Input: part model. Units: mm. Frame: model coordinates. Face numbers are marked on the shaded views. A direction names the side the tool comes from. Round coordinates to 2 decimals unless told otherwise and drop trailing zeros. Loops run counter-clockwise (first coordinate to the right, second up) from the corner with the lowest first, then second, coordinate; pieces in that order, holes last. Notation, with made-up numbers: M 28,80 L 35,80 A23 cw 35,92 Z; hole C -10,-26 d1. An arc over 180 degrees is marked long. Use one line per item in the form item = value. Start each with the question number.
Q1. Section query D-D, the plane z = -23.5. Output: boundary loops of the cut face in (x, y), and give its area (3 significant figures).
Q2. Ray query, line 1 along Y through (x, z) = (-24.5, -28.5); line 2 along Z through (x, y) = (-24, -39.5); line 3 along X through (y, z) = (-79.5, -7). Return the intervals inside material, ascending.
Q3. Access query for the marked faces 1, 2 and 3. Directions: +Z, -Z, +X, -X, +Y, -Y. A direction counts if a zero-diameter tool reaches every point of the face in a straight line with its end or side. Return the directions, or none.
Q4. Section query A-A, the plane z = -34. Output: boundary loops of the cut face in (x, y).
Q5. First-contact query: P1, Ø1.5, axis at y = -70, z = -45, coming from the +X side; P2, Ø20.5, axis at x = -74, z = -34, coming from the -Y side; P3, Ø10, axis at x = -48, z = -21, coming from the +Y side. Flat tips, straight axial feed; report the tip coordinate or a pass-through.
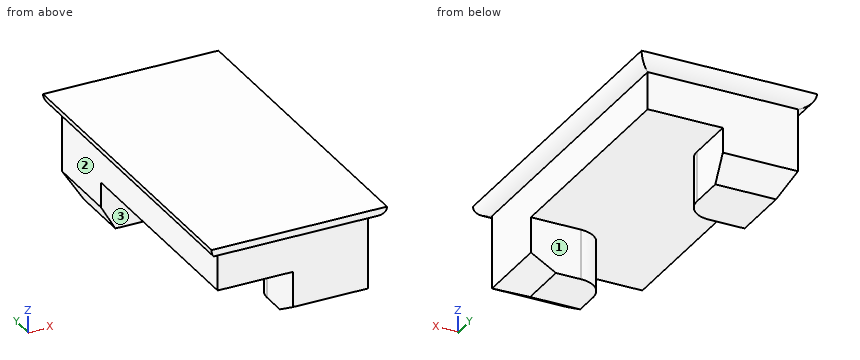
```python
from build123d import *

# Parameters (mm, degrees)
F0_W     = 88.9
F0_H     = 165.1
F1_DEPTH = 6.35
F2_DEPTH = 25.4
F3_DEPTH = 50.8
F4_R     = 6.34999
F5_SIZE2 = 7.3323484187
F5_SIZE  = 12.7
F6_SIZE2 = 7.3323484187
F6_SIZE  = 12.7


# Not quite as in the source:
# - a fillet or chamfer is up to 0.001 mm smaller than in the source, because OpenCascade refuses the exact size


with BuildPart() as f1:
    # F0 (on Top) → F1 (new body)
    with BuildSketch(Plane.XY):
        with Locations((-44.4500000971, -25.0825021148)):
            Rectangle(F0_W, F0_H)
        Polygon((-82.5500000971, 13.0174978852), (-82.5500000971, 51.1174978852), (-44.4500000971, 51.1174978852), (-6.3500000971, 51.1174978852), (-6.3500000971, -63.1825021148), (-6.3500000971, -101.2825021148), (-44.4500000971, -101.2825021148), (-82.5500000971, -101.2825021148), align=None, mode=Mode.SUBTRACT)
        with BuildLine():
            Line((-6.3500000971, 51.1174978852), (-44.4500000971, 51.1174978852))
            Line((-44.4500000971, 51.1174978852), (-44.4500000971, 25.7174978852))
            ThreePointArc((-44.4500000971, 25.7174978852), (-48.169743976, 16.7372417642), (-57.1500000971, 13.0174978852))
            Line((-57.1500000971, 13.0174978852), (-82.5500000971, 13.0174978852))
            Line((-82.5500000971, 13.0174978852), (-82.5500000971, -101.2825021148))
            Line((-82.5500000971, -101.2825021148), (-44.4500000971, -101.2825021148))
            Line((-44.4500000971, -101.2825021148), (-44.4500000971, -75.8825021148))
            ThreePointArc((-44.4500000971, -75.8825021148), (-40.7302562182, -66.9022459937), (-31.7500000971, -63.1825021148))
            Line((-31.7500000971, -63.1825021148), (-6.3500000971, -63.1825021148))
            Line((-6.3500000971, -63.1825021148), (-6.3500000971, 51.1174978852))
        make_face()
        with BuildLine():
            Line((-6.3500000971, -101.2825021148), (-6.3500000971, -63.1825021148))
            Line((-6.3500000971, -63.1825021148), (-31.7500000971, -63.1825021148))
            ThreePointArc((-31.7500000971, -63.1825021148), (-40.7302562182, -66.9022459937), (-44.4500000971, -75.8825021148))
            Line((-44.4500000971, -75.8825021148), (-44.4500000971, -101.2825021148))
            Line((-44.4500000971, -101.2825021148), (-6.3500000971, -101.2825021148))
        make_face()
        with BuildLine():
            Line((-44.4500000971, 51.1174978852), (-82.5500000971, 51.1174978852))
            Line((-82.5500000971, 51.1174978852), (-82.5500000971, 13.0174978852))
            Line((-82.5500000971, 13.0174978852), (-57.1500000971, 13.0174978852))
            ThreePointArc((-57.1500000971, 13.0174978852), (-48.169743976, 16.7372417642), (-44.4500000971, 25.7174978852))
            Line((-44.4500000971, 25.7174978852), (-44.4500000971, 51.1174978852))
        make_face()
    extrude(amount=-F1_DEPTH)

    # F0 (on Top) → F2 (join)
    with BuildSketch(Plane.XY):
        with BuildLine():
            Line((-6.3500000971, 51.1174978852), (-44.4500000971, 51.1174978852))
            Line((-44.4500000971, 51.1174978852), (-44.4500000971, 25.7174978852))
            ThreePointArc((-44.4500000971, 25.7174978852), (-48.169743976, 16.7372417642), (-57.1500000971, 13.0174978852))
            Line((-57.1500000971, 13.0174978852), (-82.5500000971, 13.0174978852))
            Line((-82.5500000971, 13.0174978852), (-82.5500000971, -101.2825021148))
            Line((-82.5500000971, -101.2825021148), (-44.4500000971, -101.2825021148))
            Line((-44.4500000971, -101.2825021148), (-44.4500000971, -75.8825021148))
            ThreePointArc((-44.4500000971, -75.8825021148), (-40.7302562182, -66.9022459937), (-31.7500000971, -63.1825021148))
            Line((-31.7500000971, -63.1825021148), (-6.3500000971, -63.1825021148))
            Line((-6.3500000971, -63.1825021148), (-6.3500000971, 51.1174978852))
        make_face()
    extrude(amount=-F2_DEPTH)

    # F0 (on Top) → F3 (join)
    with BuildSketch(Plane.XY):
        with BuildLine():
            Line((-6.3500000971, -101.2825021148), (-6.3500000971, -63.1825021148))
            Line((-6.3500000971, -63.1825021148), (-31.7500000971, -63.1825021148))
            ThreePointArc((-31.7500000971, -63.1825021148), (-40.7302562182, -66.9022459937), (-44.4500000971, -75.8825021148))
            Line((-44.4500000971, -75.8825021148), (-44.4500000971, -101.2825021148))
            Line((-44.4500000971, -101.2825021148), (-6.3500000971, -101.2825021148))
        make_face()
        with BuildLine():
            Line((-44.4500000971, 51.1174978852), (-82.5500000971, 51.1174978852))
            Line((-82.5500000971, 51.1174978852), (-82.5500000971, 13.0174978852))
            Line((-82.5500000971, 13.0174978852), (-57.1500000971, 13.0174978852))
            ThreePointArc((-57.1500000971, 13.0174978852), (-48.169743976, 16.7372417642), (-44.4500000971, 25.7174978852))
            Line((-44.4500000971, 25.7174978852), (-44.4500000971, 51.1174978852))
        make_face()
    extrude(amount=-F3_DEPTH)

    # F4 (radius 6.35 in the source; OpenCascade refuses exactly that, so slightly less here)
    f4_edges = [f1.edges().sort_by_distance(p)[0] for p in [
        (-44.45, 57.467498, -6.35),
        (0, -25.082502, -6.35),
        (-44.45, -107.632502, -6.35),
        (-88.9, -25.082502, -6.35),
    ]]
    fillet(f4_edges, radius=F4_R)

    # F5
    f5_edges = [f1.edges().sort_by_distance(p)[0] for p in [
        (-6.35, -82.232502, -50.8),
        (-25.4, -101.282502, -50.8),
    ]]
    f5_side = f1.faces().sort_by_distance((-25.003958, -82.628544, -50.8))[0]
    chamfer(f5_edges, length=F5_SIZE, length2=F5_SIZE2, reference=f5_side)

    # F6
    f6_edges = [f1.edges().sort_by_distance(p)[0] for p in [
        (-82.55, 32.067498, -50.8),
        (-63.5, 51.117498, -50.8),
    ]]
    chamfer(f6_edges, length=F6_SIZE, length2=F6_SIZE2)


solid = f1.part
```
Results found:
q1.outline = M -82.55,-101.28 L -6.35,-101.28 L -6.35,51.12 L -82.55,51.12 Z
q1.area = 11,600 mm²
q2.line_1 = -101.28 to -63.18
q2.line_2 = -25.4 to 0
q2.line_3 = -82.55 to -6.35
q3.face_1 = -Z, +X, -X, +Y
q3.face_2 = -Z, -X, +Y, -Y
q3.face_3 = -Z, +X, -X, -Y
q4.outline = M -82.55,13.02 L -57.15,13.02 A12.7 ccw -44.45,25.72 L -44.45,51.12 L -82.55,51.12 Z; M -44.45,-101.28 L -6.35,-101.28 L -6.35,-63.18 L -31.75,-63.18 A12.7 ccw -44.45,-75.88 Z
q5.P1 = -7.71
q5.P2 = -101.28
q5.P3 = 51.12
